Here's how the part is built. I have some questions about the finished solid (model axes, mm). Give positions to 0.01 mm unless a question says otherwise; leave off trailing zeros. Write each loop counter-clockwise with the first axis right and the second up, starting at its lowest first coordinate (ties: lowest second). Pieces come first, ordered by that corner, then holes. Notation, with made-up numbers: (0, 81) - (57, 81) arc R31 cw to (57, 112) - close; hole circle Ø11 at (66.25, -25.5). An arc over 180 degrees is marked (long way). Use a Markdown table: item, result.
```python
from build123d import *

# Parameters (mm, degrees)
CROQUIS1_R              = 2.5
SALIENTE_EXTRUIR1_DEPTH = 3


with BuildPart() as part:
    # Croquis1 → Saliente-Extruir1 (new body)
    with BuildSketch(Plane(origin=(0, 0, 0), x_dir=(1, 0, 0), z_dir=(0, 1, 0))):
        Polygon((23, 3), (38, 3), (38, 5.896935859), (53, 5.896935859), (53, 3), (68, 3), (68, 6), (85.5, 6), (85.5, 16), (88.5, 16), (88.5, 36), (85.5, 36), (85.5, 56), (88.5, 56), (88.5, 76), (85.5, 76), (85.5, 96), (88.5, 96), (88.5, 116), (85.5, 116), (85.5, 136), (88.5, 136), (88.5, 156), (85.5, 156), (85.5, 166), (68, 166), (68, 169), (53, 169), (53, 166), (38, 166), (38, 169), (23, 169), (23, 166), (5.5, 166), (5.5, 153), (5.5, 13), (5.5, 6), (23, 6), align=None)
        with Locations(Location((37.5, 153.396935859, 0), (0, 0, 270))):
            Circle(CROQUIS1_R, mode=Mode.SUBTRACT)
    extrude(amount=SALIENTE_EXTRUIR1_DEPTH)


solid = part.part
```
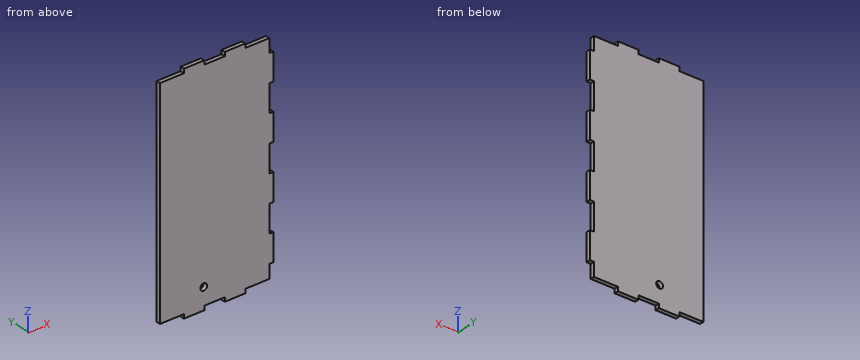
Item 1: If we section it at A-A, the plane z = -44: Write out the boundary of the cut face in (x, y).
Values:
| item | result |
|---|---|
| outline | (5.5, 0) - (85.5, 0) - (85.5, 3) - (5.5, 3) - close |
Item 2: Will these pins go through, and if not, where does the flat tip stop? pin 1 Ø0.9 at (y, z) = (1, -45) entering from +X; pin 2 Ø0.9 at (y, z) = (2, -168) entering from +X; pin 3 Ø0.9 at (y, z) = (1, -167) entering from -X; pin 4 Ø1 at (x, z) = (68, -29.5) entering from -Y.
Values:
| item | result |
|---|---|
| pin 1 | stops at x = 85.5 |
| pin 2 | stops at x = 68 |
| pin 3 | stops at x = 23 |
| pin 4 | stops at y = 0 |
Item 3: I need wall thicknesses on line 1 along Z through (x, y) = (77, 2.1); line 2 along X through (y, z) = (1.8, -121); line 3 along Z through (x, y) = (37, 1.35). Which ranges of each line are inside material? Lowest first, please. Write a range as [from, to].
Values:
| item | result |
|---|---|
| line 1 | z = [-166, -6] |
| line 2 | x = [5.5, 85.5] |
| line 3 | z = [-169, -155.85], [-150.95, -3] |
